```python
from build123d import *

# Parameters (mm, degrees)
SKETCH1_W           = 9.9
SKETCH1_H           = 6.9
BOSS_EXTRUDE1_DEPTH = 16
SKETCH2_W           = 9.9
SKETCH2_H           = 9
BOSS_EXTRUDE2_DEPTH = 10
SKETCH3_R           = 1.5
BOSS_EXTRUDE3_DEPTH = 3


with BuildPart() as part:
    # Sketch1 → Boss-Extrude1 (new body)
    with BuildSketch(Plane.XY):
        Rectangle(SKETCH1_W, SKETCH1_H)
    extrude(amount=BOSS_EXTRUDE1_DEPTH)

    # Sketch2 → Boss-Extrude2 (add)
    with BuildSketch(Plane(origin=(0, 3.45, 0), x_dir=(1, 0, 0), z_dir=(0, 1, 0))):
        with Locations((0, -4.5)):
            Rectangle(SKETCH2_W, SKETCH2_H)
    extrude(amount=BOSS_EXTRUDE2_DEPTH)

    # Sketch3 → Boss-Extrude3 (add)
    with BuildSketch(Plane(origin=(0, 0, 0), x_dir=(-1, 0, 0), z_dir=(0, 0, -1))):
        Circle(SKETCH3_R)
    extrude(amount=BOSS_EXTRUDE3_DEPTH)


solid = part.part
```
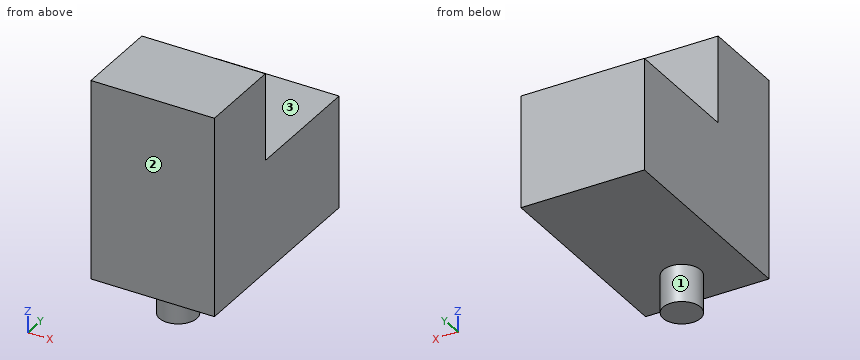
Read the model definition and answer for the solid it produces. Units are mm, in the model's axes. Face numbers are marked on the shaded views. A direction names the side the tool comes from. Coordinates: 2 decimals unless noted, no trailing zeros. Loops run counter-clockwise (first coordinate to the right, second up) from the corner with the lowest first, then second, coordinate; pieces in that order, holes last.
(1) Consider line 1 along Y through (x, z) = (-4.5, 13.25); line 2 along Z through (x, y) = (2, 5.5); line 3 along Z through (x, y) = (2, -1). Determine where each line is inside the solid, lowest interval first.
Solution:
line 1: y = -3.45 to 3.45
line 2: z = 0 to 9
line 3: z = 0 to 16
(2) The part is cut by section D-D (y = 10.5). Determine the outline of the cut face in (x, z), and give its area (3 significant figures).
Solution:
outline: (-4.95, 0) - (4.95, 0) - (4.95, 9) - (-4.95, 9) - close
area: 89.1 mm2
(3) The part is cut by section C-C (x = 2.25). Determine the outline of the cut face in (y, z).
Solution:
outline: (-3.45, 0) - (13.45, 0) - (13.45, 9) - (3.45, 9) - (3.45, 16) - (-3.45, 16) - close
(4) The part is cut by section A-A (x = 0). Determine the outline of the cut face in (y, z).
Solution:
outline: (-3.45, 0) - (-1.5, 0) - (-1.5, -3) - (1.5, -3) - (1.5, 0) - (13.45, 0) - (13.45, 9) - (3.45, 9) - (3.45, 16) - (-3.45, 16) - close
(5) A tool of negligible diameter and unlimited length cuts with its end or side. For the marked faces 1, 2 and 3, from which of +Z, -Z, +X, -X, +Y, -Y can it reach the whole face along a straight path? Write none if from no direction.
Solution:
face 1: -Z
face 2: +Z, -Z, +X, -X, -Y
face 3: +Z, +X, -X, +Y
(6) The part is cut by section B-B (y = 0). Determine the outline of the cut face in (x, z), and give its area (3 significant figures).
Solution:
outline: (-4.95, 0) - (-1.5, 0) - (-1.5, -3) - (1.5, -3) - (1.5, 0) - (4.95, 0) - (4.95, 16) - (-4.95, 16) - close
area: 167 mm2
(7) Flat-ended cylindrical pins translate along their axes: pin 1 Ø1.5 at (y, z) = (8, 11.5) entering from -X; pin 2 Ø4 at (x, y) = (-3, 9) entering from +Z; pin 3 Ø3 at (x, y) = (1, 5.5) entering from -Z; pin 4 Ø3.5 at (x, z) = (0.5, 11.5) entering from +Y. Find the tip coordinate at first contact, or state that the pin passes through.
Solution:
pin 1: passes through
pin 2: stops at z = 9
pin 3: stops at z = 0
pin 4: stops at y = 3.45
